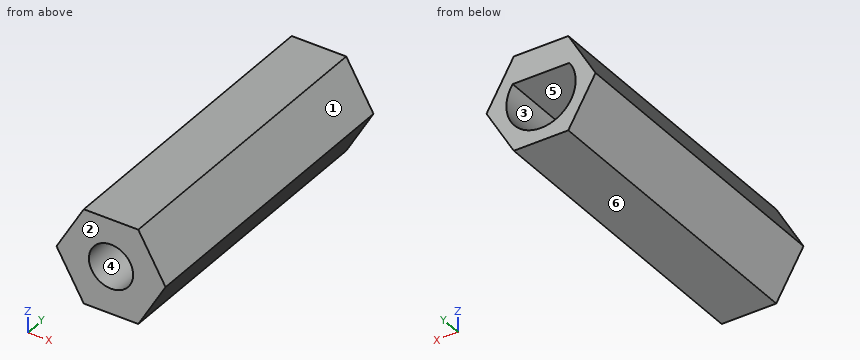
from build123d import *

# Parameters (mm, degrees)
SALIENTE_EXTRUIR1_DEPTH = 28
CORTAR_EXTRUIR1_DEPTH   = 8.3
CROQUIS3_R              = 1.5
CORTAR_EXTRUIR2_DEPTH   = 18
CROQUIS4_R              = 4
CORTAR_EXTRUIR3_DEPTH   = 7


with BuildPart() as part:
    # Croquis1 → Saliente-Extruir1 (new body)
    with BuildSketch(Plane(origin=(0, 0, 0), x_dir=(1, 0, 0), z_dir=(0, 1, 0))):
        Polygon((3.695041723, 0), (1.847520861, 3.2), (-1.847520861, 3.2), (-3.695041723, 0), (-1.847520861, -3.2), (1.847520861, -3.2), align=None)
    extrude(amount=SALIENTE_EXTRUIR1_DEPTH)

    # Croquis2 → Cortar-Extruir1 (cut)
    with BuildSketch(Plane(origin=(0, 28, 0), x_dir=(1, 0, 0), z_dir=(0, 1, 0))):
        with BuildLine():
            Line((-1.923538406, -1.35), (1.923538406, -1.35))
            ThreePointArc((1.923538406, -1.35), (0, 2.35), (-1.923538406, -1.35))
        make_face()
    extrude(amount=-CORTAR_EXTRUIR1_DEPTH, mode=Mode.SUBTRACT)

    # Croquis3 → Cortar-Extruir2 (cut)
    with BuildSketch(Plane(origin=(0, 0, 0), x_dir=(-1, 0, 0), z_dir=(0, -1, 0))):
        with Locations(Location((0, 0, 0), (0, 0, 90))):
            Circle(CROQUIS3_R)
    extrude(amount=-CORTAR_EXTRUIR2_DEPTH, mode=Mode.SUBTRACT)

    # Croquis4 → Cortar-Extruir3 (cut)
    with BuildSketch(Plane.XZ):
        Circle(CROQUIS4_R)
    extrude(amount=-CORTAR_EXTRUIR3_DEPTH, mode=Mode.SUBTRACT)


solid = part.part
Can you work these out from the model? Positions are in its coordinate system, mm. Face numbers are marked on the shaded views. A direction names the side the tool comes from. Round coordinates to 2 decimals unless told otherwise and drop trailing zeros. Write each loop counter-clockwise with the first axis right and the second up, starting at its lowest first coordinate (ties: lowest second). Pieces come first, ordered by that corner, then holes. Notation, with made-up numbers: M 55.5,72.25 L 66.5,72.25 A27 ccw 66.5,91.25 Z; hole C 63,14 d3. An arc over 180 degrees is marked long. Use CSV: the item, a comma, the result in double quotes.
(1) Imagine slicing it at D-D (y = 19.25). Write out the boundary of the cut face in (x, z).
Check values:
outline,"M -3.7,0 L -1.85,-3.2 L 1.85,-3.2 L 3.7,0 L 1.85,3.2 L -1.85,3.2 Z"
(2) I'm going to push flat-ended pins straight in: pin 1 (2 mm diameter, centred on y = 24.5, z = 1.5, fed in from +X); pin 2 (1 mm diameter, centred on y = 17, z = 1.5, fed in from +X); pin 3 (2.5 mm diameter, centred on x = 0, z = 0, fed in from -Y). Where does each tip first touch, or does it pass through?
Check values:
pin 1,"x = 3.41"
pin 2,"x = 3.12"
pin 3,"y = 18"
(3) On a 3-axis mill with a long thin cutter (end or side, diameter ignored), from which of +Z, -Z, +X, -X, +Y, -Y can I reach the whole of each face in a straight line? I mean the marked faces 4, 5 and 6. Say none if no direction works.
Check values:
face 4,"-Y"
face 5,"+Y"
face 6,"-Z, +X, -X, +Y, -Y"
(4) Imagine slicing it at C-C (z = -0.5). Write out the boundary of the cut face in (x, y).
Check values:
outline,"M -3.41,7 L -1.41,7 L -1.41,18 L 1.41,18 L 1.41,7 L 3.41,7 L 3.41,28 L 2.3,28 L 2.3,19.7 L -2.3,19.7 L -2.3,28 L -3.41,28 Z"
(5) We'd pull the mould along X, two halves only. Please class the marked faces 1, 2 and 3: +X half, -X half, draft (parallel to the pull), parting line (faces both ways), or undercut.
Check values:
face 1,"+X half"
face 2,"draft"
face 3,"undercut"
(6) I need wall thicknesses on line 1 along Y through (x, z) = (1.25, -1); line 2 along Y through (x, z) = (-1.25, 0.25); line 3 along Z through (x, y) = (0, 25). Which ranges of each line are inside material? Lowest first, please.
Check values:
line 1,"7 to 19.7"
line 2,"18 to 19.7"
line 3,"-3.2 to -2.35, 1.35 to 3.2"
(7) Imagine slicing it at A-A (y = 15.75). Write out the boundary of the cut face in (x, z), plus the area to 3 significant figures.
Check values:
outline,"M -3.7,0 L -1.85,-3.2 L 1.85,-3.2 L 3.7,0 L 1.85,3.2 L -1.85,3.2 Z; hole C 0,0 d3"
area,"28.4 mm^2"
(8) Imagine slicing it at B-B (x = 0). Write out the boundary of the cut face in (y, z).
Check values:
outline,"M 7,-3.2 L 28,-3.2 L 28,-2.35 L 19.7,-2.35 L 19.7,1.35 L 28,1.35 L 28,3.2 L 7,3.2 L 7,1.5 L 18,1.5 L 18,-1.5 L 7,-1.5 Z"
